```python
from build123d import *

# Parameters (mm, degrees)
SKETCH1_W             = 85
SKETCH1_H             = 160
BOSS_EXTRUDE1_DEPTH   = 5
SKETCH2_W             = 45
SKETCH2_H             = 65
CUT_EXTRUDE1_DEPTH    = 91.726236558
SKETCH8_W             = 57
SKETCH8_H             = 14
CUT_EXTRUDE2_DEPTH    = 91.726236558
F_2_0MM_DOWEL_HOLE1_D = 3.1
MIRROR9_COPY_1_D      = 3.1
F_2_0MM_DOWEL_HOLE3_D = 3.1
MIRROR11_COPY_1_D     = 3.1
F_2_5MM_DOWEL_HOLE4_D = 3.1
SKETCH39_W            = 85
SKETCH39_H            = 5
CUT_EXTRUDE3_DEPTH    = 35
FILLET1_R             = 10
SKETCH41_W            = 47
SKETCH41_H            = 15
SKETCH41_W_2          = 10
SKETCH41_H_2          = 45
BOSS_EXTRUDE3_DEPTH   = 4.5


with BuildPart() as part:
    # Sketch1 → Boss-Extrude1 (new body)
    with BuildSketch(Plane(origin=(0, 0, 0), x_dir=(1, 0, 0), z_dir=(0, 1, 0))):
        Rectangle(SKETCH1_W, SKETCH1_H)
    extrude(amount=BOSS_EXTRUDE1_DEPTH)

    # Sketch2 → Cut-Extrude1 (cut, through all)
    with BuildSketch(Plane(origin=(0, 5, 0), x_dir=(1, 0, 0), z_dir=(0, 1, 0))):
        Rectangle(SKETCH2_W, SKETCH2_H)
    extrude(amount=-CUT_EXTRUDE1_DEPTH, mode=Mode.SUBTRACT)

    # Sketch8 → Cut-Extrude2 (cut, through all)
    with BuildSketch(Plane(origin=(0, 5, 0), x_dir=(1, 0, 0), z_dir=(0, 1, 0))):
        with Locations((0, -80)):
            Rectangle(SKETCH8_W, SKETCH8_H)
    extrude(amount=-CUT_EXTRUDE2_DEPTH, mode=Mode.SUBTRACT)

    # Ø2.0mm Dowel Hole1 (through all)
    with Locations(Plane(origin=(26.5, 5, -30), x_dir=(0, 0, 1), z_dir=(0, 1, 0))):
        with Locations((0, 0)):
            f_2_0mm_dowel_hole1 = Hole(F_2_0MM_DOWEL_HOLE1_D / 2)

    # Mirror8: Ø2.0mm Dowel Hole1 across plane
    add(f_2_0mm_dowel_hole1.mirror(Plane(origin=(0, 0, 0), x_dir=(0, 0, 1), z_dir=(1, 0, 0))), mode=Mode.SUBTRACT)

    # Mirror9: Ø2.0mm Dowel Hole1 across plane
    add(f_2_0mm_dowel_hole1.mirror(Plane.XY), mode=Mode.SUBTRACT)

    # Mirror9 copy 1 (through all)
    with Locations(Plane(origin=(-26.5, 5, 30), x_dir=(0, 0, -1), z_dir=(0, 1, 0))):
        with Locations((0, 0)):
            Hole(MIRROR9_COPY_1_D / 2)

    # Ø2.0mm Dowel Hole3 (through all)
    with Locations(Plane(origin=(19.5, 5, -36.5), x_dir=(0, 0, 1), z_dir=(0, 1, 0))):
        with Locations((0, 0)):
            f_2_0mm_dowel_hole3 = Hole(F_2_0MM_DOWEL_HOLE3_D / 2)

    # Mirror10: Ø2.0mm Dowel Hole3 across plane
    add(f_2_0mm_dowel_hole3.mirror(Plane(origin=(0, 0, 0), x_dir=(0, 0, 1), z_dir=(1, 0, 0))), mode=Mode.SUBTRACT)

    # Mirror11: Ø2.0mm Dowel Hole3 across plane
    add(f_2_0mm_dowel_hole3.mirror(Plane.XY), mode=Mode.SUBTRACT)

    # Mirror11 copy 1 (through all)
    with Locations(Plane(origin=(-19.5, 5, 36.5), x_dir=(0, 0, -1), z_dir=(0, 1, 0))):
        with Locations((0, 0)):
            Hole(MIRROR11_COPY_1_D / 2)

    # Ø2.5mm Dowel Hole4 (through all)
    with Locations(Plane(origin=(34.5, 5, 72.5), x_dir=(0, 0, 1), z_dir=(0, 1, 0))):
        with Locations((0, 0)):
            f_2_5mm_dowel_hole4 = Hole(F_2_5MM_DOWEL_HOLE4_D / 2)

    # Mirror12: Ø2.5mm Dowel Hole4 across plane
    add(f_2_5mm_dowel_hole4.mirror(Plane(origin=(0, 0, 0), x_dir=(0, 0, 1), z_dir=(1, 0, 0))), mode=Mode.SUBTRACT)

    # Sketch39 → Cut-Extrude3 (cut)
    with BuildSketch(Plane(origin=(0, 0, -80), x_dir=(-1, 0, 0), z_dir=(0, 0, -1))):
        with Locations((0, 2.5)):
            Rectangle(SKETCH39_W, SKETCH39_H)
    extrude(amount=-CUT_EXTRUDE3_DEPTH, mode=Mode.SUBTRACT)

    # Fillet1
    fillet1_edges = [part.edges().sort_by_distance(p)[0] for p in [
        (-42.5, 2.5, -45),
        (42.5, 2.5, -45),
        (42.5, 2.5, 80),
        (-42.5, 2.5, 80),
    ]]
    fillet(fillet1_edges, radius=FILLET1_R)

    # Sketch41 → Boss-Extrude3 (add)
    with BuildSketch(Plane(origin=(0, 0, 0), x_dir=(-1, 0, 0), z_dir=(0, -1, 0))):
        with Locations((0, -55.5)):
            Rectangle(SKETCH41_W, SKETCH41_H)
        with Locations((32.5, 0)):
            Rectangle(SKETCH41_W_2, SKETCH41_H_2)
        with Locations((-32.5, 0)):
            Rectangle(SKETCH41_W_2, SKETCH41_H_2)
    extrude(amount=BOSS_EXTRUDE3_DEPTH)


solid = part.part
```
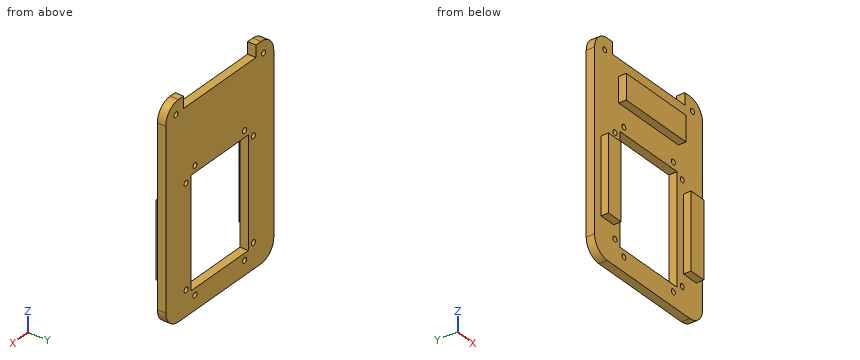
The model under review builds one solid part; all positions refer to its coordinate system, in mm. Give positions to 0.01 mm unless a question says otherwise; leave off trailing zeros. Write each loop counter-clockwise with the first axis right and the second up, starting at its lowest first coordinate (ties: lowest second). Pieces come first, ordered by that corner, then holes. Notation, with made-up numbers: M -23,-25.5 L -16,-25.5 A13 cw -16,-19.5 Z; hole C 71.5,74.25 d6. An arc over 180 degrees is marked long. Write each question's results on one line, items separated by ' | '. Start each with the question number.
1. We need section D-D (z = -15). Write out the cut boundary in (x, y).
2. We need section C-C (y = -3). Write out the cut boundary in (x, z), and give its area (4 significant figures).
3. We need section A-A (x = -1.5). Write out the cut boundary in (y, z), and give its area (4 significant figures).
4. Insertion check: pin 1 Ø1.3 at (x, y) = (31.5, -1) entering from -Z; pin 2 Ø2.5 at (x, y) = (7.5, 2) entering from +Z; pin 3 Ø2 at (y, z) = (-3, -5.5) entering from -X. Each pin has a flat end and moves straight along its axis. Give the tip position at first contact, or say it passes through.
5. For probe 1 along X at (y, z) = (3.75, -30); probe 2 along X at (y, z) = (-2.5, -8); probe 3 along X at (y, z) = (2.7, -36.5), list the stretches that pass through material, from the lowest coordinate up. Write a range as [from, to].
6. We need section B-B (z = -30). Write out the cut boundary in (x, y), and give its area (3 significant figures).
Results found:
1) outline: M -42.5,0 L -37.5,0 L -37.5,-4.5 L -27.5,-4.5 L -27.5,0 L -22.5,0 L -22.5,5 L -42.5,5 Z; M 22.5,0 L 27.5,0 L 27.5,-4.5 L 37.5,-4.5 L 37.5,0 L 42.5,0 L 42.5,5 L 22.5,5 Z
2) outline: M -37.5,-22.5 L -27.5,-22.5 L -27.5,22.5 L -37.5,22.5 Z; M -23.5,48 L 23.5,48 L 23.5,63 L -23.5,63 Z; M 27.5,-22.5 L 37.5,-22.5 L 37.5,22.5 L 27.5,22.5 Z | area: 1,605 mm^2
3) outline: M -4.5,48 L 0,48 L 0,32.5 L 5,32.5 L 5,73 L 0,73 L 0,63 L -4.5,63 Z; M 0,-45 L 5,-45 L 5,-32.5 L 0,-32.5 Z | area: 332.5 mm^2
4) pin 1: stops at z = -22.5 | pin 2: stops at z = 73 | pin 3: stops at x = -37.5
5) probe 1: x = [-42.5, -28.05], [-24.95, -22.5], [22.5, 24.95], [28.05, 42.5] | probe 2: x = [-37.5, -27.5], [27.5, 37.5] | probe 3: x = [-42.39, -21.05], [-17.95, 17.95], [21.05, 42.39]
6) outline: M -42.5,0 L -28.05,0 L -28.05,5 L -42.5,5 Z; M -24.95,0 L -22.5,0 L -22.5,5 L -24.95,5 Z; M 22.5,0 L 24.95,0 L 24.95,5 L 22.5,5 Z; M 28.05,0 L 42.5,0 L 42.5,5 L 28.05,5 Z | area: 169 mm^2
